The model under review builds one solid part; all positions refer to its coordinate system, in mm. A direction names the side the tool comes from. Round coordinates to 2 decimals unless told otherwise and drop trailing zeros. Write each loop counter-clockwise with the first axis right and the second up, starting at its lowest first coordinate (ties: lowest second). Pieces come first, ordered by that corner, then holes. Notation, with made-up numbers: (80, 74.25) -> (136, 74.25) arc R23 cw to (136, 110.25) -> close; hole circle Ø5 at (75, -28). An arc over 180 degrees is marked (long way). Answer as a JSON object with one key per item and string values. Group by question number.
1) Insertion check: pin 1 Ø8 at (y, z) = (12.5, -114) entering from +X; pin 2 Ø5.5 at (y, z) = (10.5, -183) entering from -X; pin 3 Ø5.5 at (y, z) = (10.5, -419.5) entering from -X (3 decimals). Each pin has a flat end and moves straight along its axis. Give the tip position at first contact, or say it passes through.
2) We need section C-C, the plane y = 13. Count the separate pieces of the cut face and the enclosed holes in it, then the cut area to 3 significant figures.
3) To check wall thickness, follow probe 1 along Z at (x, y) = (304.5, 9.25); probe 2 along X at (y, z) = (14.25, 6.35); probe 3 along Z at (x, y) = (256.5, 6.5). State the ranges of each line that lie inside material, in increasing order. Write a range as [from, to].
4) Mouldability with a two-part tool opening along X and no side actions: class faces 5 (the flat face through (300, 0, -177)), 6 (the flat face through (473.075, 9, -415)), 7 (the flat face through (0, 9, -105)), 8 (the cylindrical face through (50.993, 9.392, 2.424)) as pulls with the +X half, pulls with the -X half, needs draft (parallel to the pull), parting line crosses it, or undercut.
5) We need section A-A, the plane x = 406.4. Write out the cut boundary in (y, z), then the cut area to 3 significant figures.
6) We need section B-B, the plane x = 552.45. Write out the cut boundary in (y, z).
7) Machinability: for faces 1 (the flat face through (-10, 9, -133.35)), 2 (the flat face through (619, 9, -133.35)), 3 (the flat face through (151, 10, -361.95)), 4 (the flat face through (609.6, 9, -25)), which of the approach directions +Z, -Z, +X, -X, +Y, -Y give a long, thin tool a straight path to every point of the face, cutting with its end or side? Answer none if there is none.
from build123d import *

# Parameters (mm, degrees)
SKETCH_S_R              = 7.3025
SKETCH_S_R_2            = 19.05
BOSS_EXTRUDE1_DEPTH     = 19.05
FILLET1_R               = 31.75
CUT_EXTRUDE1_DEPTH      = 778.557435178
CUT_EXTRUDE1_DEPTH_BACK = 778.557435178
SKETCH4_W               = 41.275
SKETCH4_H               = 19.05
SKETCH4_W_2             = 57.15
SKETCH4_W_3             = 28.575
CUT_EXTRUDE2_DEPTH      = 19.05
SKETCH5_W               = 95.25
SKETCH5_H               = 19.05
BOSS_EXTRUDE2_DEPTH     = 133.35
FILLET2_R               = 25.4


with BuildPart() as part:
    # Sketch s → Boss-Extrude1 (new body)
    with BuildSketch(Plane(origin=(0, 0, 0), x_dir=(1, 0, 0), z_dir=(0, 1, 0))):
        with BuildLine():
            Line((0, 50.8), (0, 0))
            Line((0, 0), (0, -31.75))
            Line((0, -31.75), (609.6, -31.75))
            Line((609.6, -31.75), (609.6, 0))
            Line((609.6, 0), (609.6, 50.8))
            ThreePointArc((609.6, 50.8), (606.425, 53.975), (609.6, 57.15))
            Line((609.6, 57.15), (628.65, 57.15))
            Line((628.65, 57.15), (628.65, 76.2))
            Line((628.65, 76.2), (609.6, 76.2))
            ThreePointArc((609.6, 76.2), (606.425, 79.375), (609.6, 82.55))
            Line((609.6, 82.55), (609.6, 127))
            ThreePointArc((609.6, 127), (606.425, 130.175), (609.6, 133.35))
            Line((609.6, 133.35), (628.65, 133.35))
            Line((628.65, 133.35), (628.65, 152.4))
            Line((628.65, 152.4), (609.6, 152.4))
            ThreePointArc((609.6, 152.4), (606.425, 155.575), (609.6, 158.75))
            Line((609.6, 158.75), (609.6, 203.2))
            ThreePointArc((609.6, 203.2), (606.425, 206.375), (609.6, 209.55))
            Line((609.6, 209.55), (628.65, 209.55))
            Line((628.65, 209.55), (628.65, 228.6))
            Line((628.65, 228.6), (609.6, 228.6))
            ThreePointArc((609.6, 228.6), (606.425, 231.775), (609.6, 234.95))
            Line((609.6, 234.95), (609.6, 279.4))
            ThreePointArc((609.6, 279.4), (606.425, 282.575), (609.6, 285.75))
            Line((609.6, 285.75), (628.65, 285.75))
            Line((628.65, 285.75), (628.65, 304.8))
            Line((628.65, 304.8), (609.6, 304.8))
            ThreePointArc((609.6, 304.8), (606.425, 307.975), (609.6, 311.15))
            Line((609.6, 311.15), (609.6, 381))
            Line((609.6, 381), (444.5, 381))
            Line((444.5, 381), (444.5, 439.42))
            ThreePointArc((444.5, 439.42), (439.292358569, 451.992358569), (426.72, 457.2))
            Line((426.72, 457.2), (304.8, 457.2))
            Line((304.8, 457.2), (182.88, 457.2))
            ThreePointArc((182.88, 457.2), (170.307641431, 451.992358569), (165.1, 439.42))
            Line((165.1, 439.42), (165.1, 381))
            Line((165.1, 381), (0, 381))
            Line((0, 381), (0, 311.15))
            ThreePointArc((0, 311.15), (3.175, 307.975), (0, 304.8))
            Line((0, 304.8), (-19.05, 304.8))
            Line((-19.05, 304.8), (-19.05, 285.75))
            Line((-19.05, 285.75), (0, 285.75))
            ThreePointArc((0, 285.75), (3.175, 282.575), (0, 279.4))
            Line((0, 279.4), (0, 234.95))
            ThreePointArc((0, 234.95), (3.175, 231.775), (0, 228.6))
            Line((0, 228.6), (-19.05, 228.6))
            Line((-19.05, 228.6), (-19.05, 209.55))
            Line((-19.05, 209.55), (0, 209.55))
            ThreePointArc((0, 209.55), (3.175, 206.375), (0, 203.2))
            Line((0, 203.2), (0, 158.75))
            ThreePointArc((0, 158.75), (3.175, 155.575), (0, 152.4))
            Line((0, 152.4), (-19.05, 152.4))
            Line((-19.05, 152.4), (-19.05, 133.35))
            Line((-19.05, 133.35), (0, 133.35))
            ThreePointArc((0, 133.35), (3.175, 130.175), (0, 127))
            Line((0, 127), (0, 82.55))
            ThreePointArc((0, 82.55), (3.175, 79.375), (0, 76.2))
            Line((0, 76.2), (-19.05, 76.2))
            Line((-19.05, 76.2), (-19.05, 57.15))
            Line((-19.05, 57.15), (0, 57.15))
            ThreePointArc((0, 57.15), (3.175, 53.975), (0, 50.8))
        make_face()
        with Locations(Location((57.15, -6.35, 0), (0, 0, 90))):
            Circle(SKETCH_S_R, mode=Mode.SUBTRACT)
        with Locations(Location((266.7, -6.35, 0), (0, 0, 90))):
            Circle(SKETCH_S_R, mode=Mode.SUBTRACT)
        with Locations(Location((342.9, -6.35, 0), (0, 0, 90))):
            Circle(SKETCH_S_R, mode=Mode.SUBTRACT)
        with Locations(Location((552.45, -6.35, 0), (0, 0, 90))):
            Circle(SKETCH_S_R, mode=Mode.SUBTRACT)
        with Locations(Location((203.2, 406.4, 0), (0, 0, 90))):
            Circle(SKETCH_S_R_2, mode=Mode.SUBTRACT)
        with Locations(Location((254, 425.45, 0), (0, 0, 90))):
            Circle(SKETCH_S_R_2, mode=Mode.SUBTRACT)
        with Locations(Location((304.8, 406.4, 0), (0, 0, 90))):
            Circle(SKETCH_S_R_2, mode=Mode.SUBTRACT)
        with Locations(Location((355.6, 425.45, 0), (0, 0, 90))):
            Circle(SKETCH_S_R_2, mode=Mode.SUBTRACT)
        with Locations(Location((406.4, 406.4, 0), (0, 0, 90))):
            Circle(SKETCH_S_R_2, mode=Mode.SUBTRACT)
    extrude(amount=BOSS_EXTRUDE1_DEPTH)

    # Fillet1
    fillet1_edges = [part.edges().sort_by_distance(p)[0] for p in [
        (609.6, 9.525, 31.75),
        (0, 9.525, 31.75),
    ]]
    fillet(fillet1_edges, radius=FILLET1_R)

    # Sketch3 → Cut-Extrude1 (cut, two sides: drawn at the far end of the back side and taken through both)
    with BuildSketch(Plane(origin=(0, 19.05, 0), x_dir=(1, 0, 0), z_dir=(0, 1, 0)).offset(-CUT_EXTRUDE1_DEPTH_BACK)):
        with BuildLine():
            Line((314.325, 131.490128061), (314.325, 141.559871939))
            ThreePointArc((314.325, 141.559871939), (314.325, 146.05), (309.834871939, 146.05))
            Line((309.834871939, 146.05), (299.765128061, 146.05))
            ThreePointArc((299.765128061, 146.05), (295.275, 146.05), (295.275, 141.559871939))
            Line((295.275, 141.559871939), (295.275, 131.490128061))
            ThreePointArc((295.275, 131.490128061), (295.275, 127), (299.765128061, 127))
            Line((299.765128061, 127), (309.834871939, 127))
            ThreePointArc((309.834871939, 127), (314.325, 127), (314.325, 131.490128061))
        make_face()
        with BuildLine():
            Line((314.325, 80.690128061), (314.325, 90.759871939))
            ThreePointArc((314.325, 90.759871939), (314.325, 95.25), (309.834871939, 95.25))
            Line((309.834871939, 95.25), (299.765128061, 95.25))
            ThreePointArc((299.765128061, 95.25), (295.275, 95.25), (295.275, 90.759871939))
            Line((295.275, 90.759871939), (295.275, 80.690128061))
            ThreePointArc((295.275, 80.690128061), (295.275, 76.2), (299.765128061, 76.2))
            Line((299.765128061, 76.2), (309.834871939, 76.2))
            ThreePointArc((309.834871939, 76.2), (314.325, 76.2), (314.325, 80.690128061))
        make_face()
        with BuildLine():
            Line((314.325, 29.890128061), (314.325, 39.959871939))
            ThreePointArc((314.325, 39.959871939), (314.325, 44.45), (309.834871939, 44.45))
            Line((309.834871939, 44.45), (299.765128061, 44.45))
            ThreePointArc((299.765128061, 44.45), (295.275, 44.45), (295.275, 39.959871939))
            Line((295.275, 39.959871939), (295.275, 29.890128061))
            ThreePointArc((295.275, 29.890128061), (295.275, 25.4), (299.765128061, 25.4))
            Line((299.765128061, 25.4), (309.834871939, 25.4))
            ThreePointArc((309.834871939, 25.4), (314.325, 25.4), (314.325, 29.890128061))
        make_face()
    extrude(amount=CUT_EXTRUDE1_DEPTH + CUT_EXTRUDE1_DEPTH_BACK, mode=Mode.SUBTRACT)

    # Sketch4 → Cut-Extrude2 (cut)
    with BuildSketch(Plane(origin=(0, 19.05, 0), x_dir=(1, 0, 0), z_dir=(0, 1, 0))):
        with Locations((20.6375, 371.475)):
            Rectangle(SKETCH4_W, SKETCH4_H)
        with Locations((88.9, 371.475)):
            Rectangle(SKETCH4_W_2, SKETCH4_H)
        with Locations((150.8125, 371.475)):
            Rectangle(SKETCH4_W_3, SKETCH4_H)
        with Locations((458.7875, 371.475)):
            Rectangle(SKETCH4_W_3, SKETCH4_H)
        with Locations((520.7, 371.475)):
            Rectangle(SKETCH4_W_2, SKETCH4_H)
        with Locations((588.9625, 371.475)):
            Rectangle(SKETCH4_W, SKETCH4_H)
    extrude(amount=-CUT_EXTRUDE2_DEPTH, mode=Mode.SUBTRACT)

    # Sketch5 → Boss-Extrude2 (add)
    with BuildSketch(Plane(origin=(0, 0, -361.95), x_dir=(-1, 0, 0), z_dir=(0, 0, -1))):
        with Locations((-520.7, 9.525)):
            Rectangle(SKETCH5_W, SKETCH5_H)
        with Locations((-88.9, 9.525)):
            Rectangle(SKETCH5_W, SKETCH5_H)
    extrude(amount=BOSS_EXTRUDE2_DEPTH)

    # Fillet2
    fillet2_edges = [part.edges().sort_by_distance(p)[0] for p in [
        (568.325, 9.525, -495.3),
        (473.075, 9.525, -495.3),
        (136.525, 9.525, -495.3),
        (41.275, 9.525, -495.3),
    ]]
    fillet(fillet2_edges, radius=FILLET2_R)


solid = part.part
Here are the results:
{
 "1": {"pin 1": "stops at x = 609.6", "pin 2": "stops at x = 0", "pin 3": "stops at x = 41.275"},
 "2": {"separate pieces": "1", "enclosed holes": "12", "area": "286,000 mm^2"},
 "3": {"probe 1": "z = [-457.2, -425.45], [-387.35, -146.05], [-127, -95.25], [-76.2, -44.45], [-25.4, 31.75]", "probe 2": "x = [0.64, 49.85], [64.45, 259.4], [274, 335.6], [350.2, 545.15], [559.75, 608.96]", "probe 3": "z = [-457.2, -444.34], [-406.56, 31.75]"},
 "4": {"face 5": "needs draft", "face 6": "undercut", "face 7": "pulls with the -X half", "face 8": "undercut"},
 "5": {"outline": "(0, -457.2) -> (19.05, -457.2) -> (19.05, -425.45) -> (0, -425.45) -> close; (0, -387.35) -> (19.05, -387.35) -> (19.05, 31.75) -> (0, 31.75) -> close", "area": "8,590 mm^2"},
 "6": {"outline": "(0, -493.45) -> (19.05, -493.45) -> (19.05, -0.95) -> (0, -0.95) -> close; (0, 13.65) -> (19.05, 13.65) -> (19.05, 31.75) -> (0, 31.75) -> close"},
 "7": {"face 1": "-X, +Y, -Y", "face 2": "+X, +Y, -Y", "face 3": "-Z, +Y, -Y", "face 4": "+Z, +X, +Y, -Y"}
}
